from build123d import *

# Parameters (mm, degrees)
EXTRUDE_2_DEPTH     = 10
SKETCH_3_R          = 1.5
EXTRUDE_3_DEPTH     = 1.5
SKETCH_5_R          = 1.65
CUT_EXTRUDE_2_DEPTH = 27.084669827
FILLET_1_R          = 6
SKETCH_6_W          = 10
SKETCH_6_H          = 1
SKETCH_6_W_2        = 5
EXTRUDE_4_DEPTH     = 4
SKETCH_7_W          = 5.689599517
SKETCH_7_H          = 3.3
CUT_EXTRUDE_3_DEPTH = 0.5
SKETCH_8_W          = 14.19653451
SKETCH_8_H          = 16.2
CUT_EXTRUDE_4_DEPTH = 30.624989451
MOVE_FACE_1_BY      = 12
CUT_EXTRUDE_5_REACH = 32.441
SKETCH_9_W          = 16.770919553
SKETCH_9_H          = 12.2
SKETCH_10_R         = 1.65
CUT_EXTRUDE_6_DEPTH = 31.127064245
FILLET_2_R          = 6
MOVE_FACE_2_BY      = 1


with BuildPart() as part:
    # Эскиз2 → Бобышка-Вытянуть2 (new body)
    with BuildSketch(Plane.XY):
        Polygon((0, 0), (0, 2), (13, 2), (13, -0.1), (24, -0.1), (24, -2.1), (11, -2.1), (11, 0), align=None)
    extrude(amount=EXTRUDE_2_DEPTH)

    # Эскиз3 → Бобышка-Вытянуть3 (add)
    with BuildSketch(Plane(origin=(0, -0.1, 0), x_dir=(1, 0, 0), z_dir=(0, 1, 0))):
        with Locations(Location((18.1, -5, 0), (0, 0, 90))):
            Circle(SKETCH_3_R)
    extrude(amount=EXTRUDE_3_DEPTH)

    # Эскиз5 → Вырез-Вытянуть2 (cut, through all)
    with BuildSketch(Plane.XZ):
        with Locations((5, 5)):
            Circle(SKETCH_5_R)
    extrude(amount=-CUT_EXTRUDE_2_DEPTH, mode=Mode.SUBTRACT)

    # Скругление1
    fillet_1_edges = [part.edges().sort_by_distance(p)[0] for p in [
        (24, -1.1, 10),
        (0, 1, 10),
    ]]
    fillet(fillet_1_edges, radius=FILLET_1_R)

    # Эскиз6 → Бобышка-Вытянуть4 (add)
    with BuildSketch(Plane(origin=(0, -2.1, 0), x_dir=(-1, 0, 0), z_dir=(0, -1, 0))):
        with Locations((-16, -0.5)):
            Rectangle(SKETCH_6_W, SKETCH_6_H)
        with Locations((-13.5, -9.5)):
            Rectangle(SKETCH_6_W_2, SKETCH_6_H)
    extrude(amount=EXTRUDE_4_DEPTH)

    # Эскиз7 → Вырез-Вытянуть3 (cut)
    with BuildSketch(Plane.XZ):
        with Locations((2.155200242, 5)):
            Rectangle(SKETCH_7_W, SKETCH_7_H)
    extrude(amount=-CUT_EXTRUDE_3_DEPTH, mode=Mode.SUBTRACT)

    # Зеркальное отражение1: part across plane


with BuildPart() as part_1:
    add(part.part)
    add(part.part.mirror(Plane.ZX.offset(-6.1)))

    # Эскиз8 → Вырез-Вытянуть4 (cut, through all)
    with BuildSketch(Plane.XY.offset(10)):
        with Locations((20.098267255, -6.1)):
            Rectangle(SKETCH_8_W, SKETCH_8_H)
    extrude(amount=-CUT_EXTRUDE_4_DEPTH, mode=Mode.SUBTRACT)

    # Move Face 1: a face moved outward by 12.0
    extrude(part_1.faces().sort_by_distance((13, -10.15, 5))[0], amount=MOVE_FACE_1_BY, dir=(1, 0, 0))

    # Вырез-Вытянуть5: up to this face of the body (flat: up to its plane)
    cut_extrude_5_end = Plane(part_1.part.faces().sort_by_distance((18, -6.1, 1))[0])
    # Эскиз9 → Вырез-Вытянуть5 (cut, up to the picked face)
    with BuildSketch(Plane.XY.offset(10), mode=Mode.PRIVATE) as cut_extrude_5_sk1:
        with Locations((21.385459776, -6.1)):
            Rectangle(SKETCH_9_W, SKETCH_9_H)
    cut_extrude_5_tool1 = split(extrude(cut_extrude_5_sk1.sketch, amount=-CUT_EXTRUDE_5_REACH, mode=Mode.PRIVATE), bisect_by=cut_extrude_5_end, keep=Keep.BOTH, mode=Mode.PRIVATE)
    add(cut_extrude_5_tool1.solids().sort_by(Axis((21.38546, -6.1, 10), (0, 0, -1)))[0], mode=Mode.SUBTRACT)

    # Эскиз10 → Вырез-Вытянуть6 (cut, through all)
    with BuildSketch(Plane.XY.offset(1)):
        with Locations((16, -9.1)):
            Circle(SKETCH_10_R)
        with Locations((22, -3.1)):
            Circle(SKETCH_10_R)
    extrude(amount=-CUT_EXTRUDE_6_DEPTH, mode=Mode.SUBTRACT)

    # Скругление2
    fillet_2_edges = [part_1.edges().sort_by_distance(p)[0] for p in [
        (25, -13.2, 10),
        (25, 1, 10),
    ]]
    fillet(fillet_2_edges, radius=FILLET_2_R)

    # Move Face 2: a face moved outward by 1.0
    extrude(part_1.faces().sort_by_distance((18.229149322, -6.1, 1))[0], amount=MOVE_FACE_2_BY, dir=(0, 0, 1))


solid = part_1.part
The listing builds one solid part. Answer for the finished solid, in the listing's coordinates (mm). A direction names the side the tool comes from. Round coordinates to 2 decimals unless told otherwise and drop trailing zeros. Loops run counter-clockwise (first coordinate to the right, second up) from the corner with the lowest first, then second, coordinate; pieces in that order, holes last. Notation, with made-up numbers: M 53.5,36 L 74.5,36 A34 cw 74.5,69 Z; hole C -35,71 d5. An arc over 180 degrees is marked long. Return JSON: item names as keys, results as strings.
Q1. Find section B-B, the plane x = 16. Determine the outline of the cut face in (y, z).
Results list:
{"outline": "M -14.2,0 L -10.75,0 L -10.75,2 L -12.2,2 L -12.2,10 L -14.2,10 Z; M -7.45,0 L 2,0 L 2,10 L 0,10 L 0,2 L -7.45,2 Z"}
Q2. Find section D-D, the plane z = 5.75. Determine the outline of the cut face in (x, y).
Results list:
{"outline": "M 0.26,-14.2 L 3.53,-14.2 L 3.53,-12.7 L 0.26,-12.7 Z; M 0.26,0.5 L 3.53,0.5 L 3.53,2 L 0.26,2 Z; M 6.47,-14.2 L 24.74,-14.2 L 24.74,-12.2 L 13,-12.2 L 13,-10.1 L 11,-10.1 L 11,-12.2 L 6.47,-12.2 Z; M 6.47,0 L 11,0 L 11,-2.1 L 13,-2.1 L 13,0 L 24.74,0 L 24.74,2 L 6.47,2 Z"}
Q3. Find section A-A, the plane z = 3. Determine the outline of the cut face in (x, y).
Results list:
{"outline": "M 0,-14.2 L 25,-14.2 L 25,-12.2 L 13,-12.2 L 13,-10.1 L 11,-10.1 L 11,-12.2 L 0,-12.2 Z; M 0,0 L 11,0 L 11,-2.1 L 13,-2.1 L 13,0 L 25,0 L 25,2 L 0,2 Z"}
Q4. The mould has two halves that part along Y. Classify faces 1 (the face through (0, -13, 2)), 2 (the face through (19, 0, 6)), 3 (the face through (12, -14.2, 5)): released by +Y, released by -Y, zero draft, split by the parting line, or undercut.
Results list:
{"face 1": "zero draft", "face 2": "undercut", "face 3": "released by -Y"}
Q5. Which of the six approach directions +Z, -Z, +X, -X, +Y, -Y give full straight-line access (tool end or side, diameter ignored) to faces 4 (the face through (2, -12.7, 5)), 5 (the face through (11, -6, 1.6)), 6 (the face through (12, -6, 9)), 7 (the face through (6.524, 0.986, 4.368)), 8 (the face through (13, -7.5, 9.6))?
Results list:
{"face 4": "-X", "face 5": "+Z, -Z, -X", "face 6": "+X, -X", "face 7": "+Y, -Y", "face 8": "+Z, +X"}
Q6. Find the intervals of material crossed by line 1 along Y through (x, z) = (15.25, 3.75); line 2 along Y through (x, z) = (2.75, 6.5); line 3 along X through (y, z) = (-4.5, 9.5), in increasing order. Write a range as from..to.
Results list:
{"line 1": "y = -14.2..-12.2, 0..2", "line 2": "y = -14.2..-12.7, 0.5..2", "line 3": "x = 11..13"}
Q7. Find section C-C, the plane y = -3.1. Determine the outline of the cut face in (x, z).
Results list:
{"outline": "M 11,0 L 20.35,0 L 20.35,2 L 11,2 Z; M 11,9 L 13,9 L 13,10 L 11,10 Z; M 23.65,0 L 25,0 L 25,2 L 23.65,2 Z"}
Q8. Each of these flat-tipped pins is pushed along its axis until it touches: pin 1 Ø3.5 at (x, y) = (18.5, -6.5) entering from +Z; pin 2 Ø3 at (x, z) = (5, 5) entering from -Y; pin 3 Ø3 at (y, z) = (-7, 2.5) entering from -X. Where does it stop, or does it pass through?
Results list:
{"pin 1": "stops at z = 2", "pin 2": "passes through", "pin 3": "stops at x = 11"}
